```python
from build123d import *

# Parameters (mm, degrees)
SKETCH1_W                = 40
SKETCH1_H                = 60
BOSS_EXTRUDE1_DEPTH      = 1.6
BOSS_EXTRUDE2_DEPTH      = 5.4
BOSS_EXTRUDE2_DEPTH_BACK = 3
SKETCH2_W                = 18.5
SKETCH2_H                = 4.5


with BuildPart() as part:
    # Sketch1 → Boss-Extrude1 (new body)
    with BuildSketch(Plane(origin=(0, 0, 0), x_dir=(0, 1, 0), z_dir=(0, 0, 1))):
        Rectangle(SKETCH1_W, SKETCH1_H)
    extrude(amount=BOSS_EXTRUDE1_DEPTH)

    # Sketch2 → Boss-Extrude2 (add, two sides: drawn at the far end of the back side and taken through both)
    with BuildSketch(Plane.YZ.offset(30).offset(-BOSS_EXTRUDE2_DEPTH_BACK)):
        with Locations((0, 3.85)):
            Rectangle(SKETCH2_W, SKETCH2_H)
    extrude(amount=BOSS_EXTRUDE2_DEPTH + BOSS_EXTRUDE2_DEPTH_BACK)


solid = part.part
```
Could you check a few things on this model? Use its own coordinates, in mm. A direction names the side the tool comes from. Round coordinates to 2 decimals unless told otherwise and drop trailing zeros. Loops run counter-clockwise (first coordinate to the right, second up) from the corner with the lowest first, then second, coordinate; pieces in that order, holes last.
Q1. On a 3-axis mill with a long thin cutter (end or side, diameter ignored), from which of +Z, -Z, +X, -X, +Y, -Y can I reach the whole of each face in a straight line? I mean faces 1 (the flat face through (31, -9.25, 4)), 2 (the flat face through (31, 9.25, 4)), 3 (the flat face through (0, 0, 0)), 4 (the flat face through (30, 0, 1)), 5 (the flat face through (27, 0, 4)). Say none if no direction works.
Q2. I want a section at B-B (z = 3). Write out the boundary of the cut face in (x, y).
Q3. I want a section at C-C (x = 18.5). Write out the boundary of the cut face in (y, z), and give its area (3 significant figures).
Q4. For P1, Ø2.5, axis at x = 34, y = -1.5, coming from the -Z side; P2, Ø10, axis at x = 0.5, y = -13.5, coming from the +Z side; P3, Ø1.3, axis at x = 33, z = 4.5, coming from the -Y side, each with a flat end and sliding along its axis, tell me the tip position at first contact or that it passes through.
Q5. Please list where these lines run through material, in increasing order: L1, parallel to Z at x = -2.5, y = -10; L2, parallel to X at y = 3, z = 2; L3, parallel to X at y = 13, z = 0.5.
Q6. I want a section at A-A (y = 0). Write out the boundary of the cut face in (x, z), and give its area (3 significant figures).
Answer below:
1. face 1: +Z, +X, -X, -Y
1. face 2: +Z, +X, -X, +Y
1. face 3: -Z, +X, -X, +Y, -Y
1. face 4: -Z, +X, +Y, -Y
1. face 5: +Z, -X, +Y, -Y
2. outline: (27, -9.25) - (35.4, -9.25) - (35.4, 9.25) - (27, 9.25) - close
3. outline: (-20, 0) - (20, 0) - (20, 1.6) - (-20, 1.6) - close
3. area: 64.0 mm2
4. P1: stops at z = 1.6
4. P2: stops at z = 1.6
4. P3: stops at y = -9.25
5. L1: z = 0 to 1.6
5. L2: x = 27 to 35.4
5. L3: x = -30 to 30
6. outline: (-30, 0) - (30, 0) - (30, 1.6) - (35.4, 1.6) - (35.4, 6.1) - (27, 6.1) - (27, 1.6) - (-30, 1.6) - close
6. area: 134 mm2
